Could you check a few things on this model? Use its own coordinates, in mm. A direction names the side the tool comes from. Give positions to 0.01 mm unless a question says otherwise; leave off trailing zeros. Order: outer loops, then holes, each group sorted by start corner. A loop starts at its lowest first (then second) coordinate and runs counter-clockwise, first axis right, second up. Notation, with made-up numbers: (-5, 30) -> (47, 30) arc R20 cw to (47, 48) -> close; hole circle Ø6 at (43.25, 30.5). An arc over 180 degrees is marked (long way). Use one line per item in the form item = value. Start each with the question number.
from build123d import *

# Parameters (mm, degrees)
SALIENTE_EXTRUIR1_DEPTH      = 4
SALIENTE_EXTRUIR1_DEPTH_BACK = 1
CROQUIS4_R                   = 6
CORTAR_EXTRUIR1_DEPTH        = 1.5
CROQUIS8_R                   = 2.4
CORTAR_EXTRUIR2_DEPTH        = 2.4
CORTAR_EXTRUIR3_REACH        = 4.6
CROQUIS9_R                   = 1.1
CROQUIS10_R                  = 12.5
CROQUIS10_R_2                = 9.5
EXTRUIR_L_MINA1_DEPTH        = 5
CORTAR_EXTRUIR4_DEPTH        = 0.3


with BuildPart() as part:
    # Croquis1 → Saliente-Extruir1 (new body, two sides)
    with BuildSketch(Plane(origin=(0, 0, 0), x_dir=(1, 0, 0), z_dir=(0, 1, 0))) as saliente_extruir1_sk:
        with BuildLine():
            Line((-14, 20), (14, 20))
            ThreePointArc((14, 20), (18.242640687, 18.242640687), (20, 14))
            Line((20, 14), (20, -14))
            ThreePointArc((20, -14), (18.242640687, -18.242640687), (14, -20))
            Line((14, -20), (-14, -20))
            ThreePointArc((-14, -20), (-18.242640687, -18.242640687), (-20, -14))
            Line((-20, -14), (-20, 14))
            ThreePointArc((-20, 14), (-18.242640687, 18.242640687), (-14, 20))
        make_face()
    extrude(amount=SALIENTE_EXTRUIR1_DEPTH)
    extrude(saliente_extruir1_sk.sketch, amount=-SALIENTE_EXTRUIR1_DEPTH_BACK)

    # Croquis4 → Cortar-Extruir1 (cut)
    with BuildSketch(Plane.XZ.offset(1)):
        Circle(CROQUIS4_R)
    extrude(amount=-CORTAR_EXTRUIR1_DEPTH, mode=Mode.SUBTRACT)

    # Croquis8 → Cortar-Extruir2 (cut)
    with BuildSketch(Plane(origin=(0, 4, 0), x_dir=(1, 0, 0), z_dir=(0, 1, 0))):
        Circle(CROQUIS8_R)
    extrude(amount=-CORTAR_EXTRUIR2_DEPTH, mode=Mode.SUBTRACT)

    # Croquis9 → Cortar-Extruir3 (cut, up to next)
    with BuildSketch(Plane(origin=(0, 1.6, 0), x_dir=(1, 0, 0), z_dir=(0, 1, 0)), mode=Mode.PRIVATE) as cortar_extruir3_sk1:
        Circle(CROQUIS9_R)
    cortar_extruir3_tool1 = extrude(cortar_extruir3_sk1.sketch, amount=-CORTAR_EXTRUIR3_REACH, mode=Mode.PRIVATE) & part.part
    add(cortar_extruir3_tool1.solids().sort_by_distance((0, 1.6, 0))[0], mode=Mode.SUBTRACT)

    # Croquis10 → Extruir-Lámina1 (add)
    with BuildSketch(Plane(origin=(0, 4, 0), x_dir=(1, 0, 0), z_dir=(0, 1, 0))):
        Circle(CROQUIS10_R)
        Circle(CROQUIS10_R_2, mode=Mode.SUBTRACT)
    extrude(amount=EXTRUIR_L_MINA1_DEPTH)

    # Croquis11 → Cortar-Extruir4 (cut)
    with BuildSketch(Plane(origin=(0, 4, 0), x_dir=(1, 0, 0), z_dir=(0, 1, 0))):
        Polygon((-14, 11.5), (-14, 12.2), (-15, 12.2), (-15, 16.5), (-15.7, 16.5), (-15.7, 11.5), align=None)
        Polygon((-12.3, 16.5), (-14, 16.5), (-14, 15.8), (-13, 15.8), (-13, 11.5), (-12.3, 11.5), align=None)
    extrude(amount=-CORTAR_EXTRUIR4_DEPTH, mode=Mode.SUBTRACT)


solid = part.part
(1) Imagine slicing it at B-B (x = 0). Write out the boundary of the cut face in (y, z).
(2) Imagine slicing it at A-A (z = 0). Write out the boundary of the cut face in (x, y), plus the area to 3 significant figures.
(3) Imagine slicing it at C-C (y = 3). Write out the boundary of the cut face in (x, z).
(4) Imagine slicing it at D-D (x = 5.5). Write out the boundary of the cut face in (y, z).
(5) Which directions (+Z, -Z, +X, -X, +Y, -Y) give clear straight access to the entire face, cutting with the end or side of a thin tool? Please do faces 1 (the cylindrical face through (1.29, 2.817, -2.024)), 2 (the cylindrical face through (18.196, 1.535, -18.289)), 3 (the flat face through (1.25, 0.5, 0.08)).
(6) I'm going to push flat-ended pins straight in: pin 1 Ø2.5 at (x, z) = (0.5, 0) entering from +Y; pin 2 Ø4 at (x, z) = (11, 10) entering from +Y; pin 3 Ø3 at (y, z) = (7, -0.5) entering from -X. Where does each tip first touch, or does it pass through?
(7) We'd pull the mould along X, two halves only. Please class faces 4 (the flat face through (1, 1.6, -1)), 5 (the cylindrical face through (18.289, 1.535, 18.196)), 6 (the flat face through (0, 2, -20)): pulls with the +X half, pulls with the -X half, needs draft (parallel to the pull), parting line crosses it, or undercut.
(8) Please list where these lines run through material, in increasing order: probe 1 along Z at (x, y) = (0, 3.5); probe 2 along Z at (x, y) = (0, -0.45); probe 3 along X at (y, z) = (5.1, 0).
Calculated:
q1.outline = (-1, -20) -> (4, -20) -> (4, -12.5) -> (9, -12.5) -> (9, -9.5) -> (4, -9.5) -> (4, -2.4) -> (1.6, -2.4) -> (1.6, -1.1) -> (0.5, -1.1) -> (0.5, -6) -> (-1, -6) -> close; (-1, 6) -> (0.5, 6) -> (0.5, 1.1) -> (1.6, 1.1) -> (1.6, 2.4) -> (4, 2.4) -> (4, 9.5) -> (9, 9.5) -> (9, 12.5) -> (4, 12.5) -> (4, 20) -> (-1, 20) -> close
q2.outline = (-20, -1) -> (-6, -1) -> (-6, 0.5) -> (-1.1, 0.5) -> (-1.1, 1.6) -> (-2.4, 1.6) -> (-2.4, 4) -> (-9.5, 4) -> (-9.5, 9) -> (-12.5, 9) -> (-12.5, 4) -> (-20, 4) -> close; (1.1, 0.5) -> (6, 0.5) -> (6, -1) -> (20, -1) -> (20, 4) -> (12.5, 4) -> (12.5, 9) -> (9.5, 9) -> (9.5, 4) -> (2.4, 4) -> (2.4, 1.6) -> (1.1, 1.6) -> close
q2.area = 198 mm2
q3.outline = (-20, -14) arc R6 ccw to (-14, -20) -> (14, -20) arc R6 ccw to (20, -14) -> (20, 14) arc R6 ccw to (14, 20) -> (-14, 20) arc R6 ccw to (-20, 14) -> close; hole circle Ø4.8 at (0, 0)
q4.outline = (-1, -20) -> (4, -20) -> (4, -11.22) -> (9, -11.22) -> (9, -7.75) -> (4, -7.75) -> (4, 7.75) -> (9, 7.75) -> (9, 11.22) -> (4, 11.22) -> (4, 20) -> (-1, 20) -> (-1, 2.4) -> (0.5, 2.4) -> (0.5, -2.4) -> (-1, -2.4) -> close
q5.face_1 = +Y
q5.face_2 = -Z, +X, +Y, -Y
q5.face_3 = -Y
q6.pin_1 = 1.6
q6.pin_2 = 4
q6.pin_3 = -12.5
q7.face_4 = undercut
q7.face_5 = pulls with the +X half
q7.face_6 = needs draft
q8.probe_1 = -20 to -2.4, 2.4 to 20
q8.probe_2 = -20 to -6, 6 to 20
q8.probe_3 = -12.5 to -9.5, 9.5 to 12.5
